from build123d import *

# Parameters (mm, degrees)
F1_DEPTH = 27.5
F2_R     = 5
F3_R     = 0.5
F5_D     = 5.5


with BuildPart() as f1:
    # F0 (on Front) → F1 (new body, symmetric)
    with BuildSketch(Plane.XZ):
        Polygon((-7.5, 0), (0, 0), (7.5, 0), (7.5, 38.8618100292), (5, 38.8618100292), (5, 2.5), (-5, 2.5), (-5, 38.8618100292), (-7.5, 38.8618100292), align=None)
    extrude(amount=F1_DEPTH, both=True)

    # F2
    f2_edges = [f1.edges().sort_by_distance(p)[0] for p in [
        (6.25, -27.5, 38.86181),
        (-6.25, -27.5, 38.86181),
        (6.25, 27.5, 38.86181),
        (-6.25, 27.5, 38.86181),
    ]]
    fillet(f2_edges, radius=F2_R)

    # F3
    f3_edges = [f1.edges().sort_by_distance(p)[0] for p in [
        (-5, 0, 2.5),
        (5, 0, 2.5),
    ]]
    fillet(f3_edges, radius=F3_R)

    # F5 (through all)
    with Locations(Plane.XY.offset(2.5)):
        with Locations((0, 17.5), (0, -17.5)):
            Hole(F5_D / 2)


solid = f1.part
Geometry: final body of the model. Coordinates: model frame, mm. A direction names the side the tool comes from. Round coordinates to 2 decimals unless told otherwise and drop trailing zeros. Order: outer loops, then holes, each group sorted by start corner. A loop starts at its lowest first (then second) coordinate and runs counter-clockwise, first axis right, second up.
Q1. Section A-A, the plane z = 10.5. Output: boundary loops of the cut face in (x, y), and give its area (3 significant figures).
Result sheet:
outline: (-7.5, -27.5) - (-5, -27.5) - (-5, 27.5) - (-7.5, 27.5) - close; (5, -27.5) - (7.5, -27.5) - (7.5, 27.5) - (5, 27.5) - close
area: 275 mm2
Q2. Section D-D, the plane y = -9. Output: boundary loops of the cut face in (x, z), and give its area (3 significant figures).
Result sheet:
outline: (-7.5, 0) - (7.5, 0) - (7.5, 38.86) - (5, 38.86) - (5, 3) arc R0.5 cw to (4.5, 2.5) - (-4.5, 2.5) arc R0.5 cw to (-5, 3) - (-5, 38.86) - (-7.5, 38.86) - close
area: 219 mm2
Q3. Access query for faces 1 (the face through (5, 0, 21)), 2 (the face through (-7, -27.5, 13)). Directions: +Z, -Z, +X, -X, +Y, -Y. A direction counts if a zero-diameter tool reaches every point of the face in a straight line with its end or side. Return the directions, or none.
Result sheet:
face 1: +Z, +Y, -Y
face 2: +Z, -Z, +X, -X, -Y
Q4. Material intervals for probe 1 along Y at (x, z) = (0, 0.6); probe 2 along X at (y, z) = (-18, 22.5); probe 3 along Z at (x, y) = (-3.5, 2), sorted ascending.
Result sheet:
probe 1: y = -27.5 to -20.25, -14.75 to 14.75, 20.25 to 27.5
probe 2: x = -7.5 to -5, 5 to 7.5
probe 3: z = 0 to 2.5
Q5. Section C-C, the plane y = 17.5. Output: boundary loops of the cut face in (x, z), and give its area (3 significant figures).
Result sheet:
outline: (-7.5, 0) - (-2.75, 0) - (-2.75, 2.5) - (-4.5, 2.5) arc R0.5 cw to (-5, 3) - (-5, 38.86) - (-7.5, 38.86) - close; (2.75, 0) - (7.5, 0) - (7.5, 38.86) - (5, 38.86) - (5, 3) arc R0.5 cw to (4.5, 2.5) - (2.75, 2.5) - close
area: 206 mm2
Q6. Pin query (flat end, axial travel): pin 1 (6.5 mm diameter, centred on x = 0, y = -17.5, fed in from -Z); pin 2 (9 mm diameter, centred on x = 0, y = 17.5, fed in from +Z). Return the tip coordinate at first contact, or that it passes through.
Result sheet:
pin 1: stops at z = 0
pin 2: stops at z = 2.5
Q7. Mould query, pull axis Y, two halves, no side actions, for faces 3 (the face through (-6.268, -25.996, 37.436)), 4 (the face through (0.358, 20.227, 1.233)), 5 (the face through (-6.268, 25.996, 37.436)). Classes: released by +Y, released by -Y, zero draft, split by the parting line, or undercut.
Result sheet:
face 3: released by -Y
face 4: undercut
face 5: released by +Y
Q8. Section B-B, the plane x = 0. Output: boundary loops of the cut face in (y, z), and give its area (3 significant figures).
Result sheet:
outline: (-27.5, 0) - (-20.25, 0) - (-20.25, 2.5) - (-27.5, 2.5) - close; (-14.75, 0) - (14.75, 0) - (14.75, 2.5) - (-14.75, 2.5) - close; (20.25, 0) - (27.5, 0) - (27.5, 2.5) - (20.25, 2.5) - close
area: 110 mm2
